Verification items for this drawing (mm, ordinates from the low corner). A direction names the side the tool comes from. Coordinates: 2 decimals unless noted, no trailing zeros. Order: outer loops, then holes, each group sorted by start corner. A loop starts at its lowest first (then second) coordinate and runs counter-clockwise, first axis right, second up. Notation, with made-up numbers: M -39,44 L -35,44 A4 cw -35,51 Z; hole C 53,16.5 d6. An arc over 180 degrees is marked long. One line per item, written item: value. Start each with the question number.
1) Access from +Z, -Z, +X, -X, +Y, -Y to the whole of each face (thin tool, end or side, straight path). Record for the marked faces 4, 5 and 6.
2) Draft check along Y on the marked faces 1, 2 and 3. Enter one of: pulls with the +Y half, pulls with the -Y half, needs draft (parallel to the pull), parting line crosses it, or undercut.
3) Go/stop test with flat-tipped pins: P1, Ø1.6, axis at y = 48, z = 5.5, coming from the -X side; P2, Ø4, axis at y = 41.5, z = 5, coming from the -X side; P3, Ø4.5, axis at x = 13.5, z = 6.5, coming from the +Y side; P4, Ø4, axis at x = 5, y = 28.5, coming from the -Z side. Record where each tip stops, or that it passes through.
4) Sectioned sample at A-A, the plane x = 28. Enter the section's corners in (y, z), then the cut area to 4 significant figures.
5) Sectioned sample at D-D, the plane x = 8. Enter the section's corners in (y, z), then the cut area to 3 significant figures.
6) Sectioned sample at C-C, the plane z = 9.25. Enter the section's corners in (x, y).
7) Sectioned sample at B-B, the plane y = 13. Enter the section's corners in (x, z), then the cut area to 3 significant figures.
8) Thickness scan on L1, parallel to Y at x = 24.5, z = 9.25; L2, parallel to X at y = 12.5, z = 7.25; L3, parallel to Y at x = 9.5, z = 10.5. Record the ranges inside material, lowest first. Write a range as from..to.
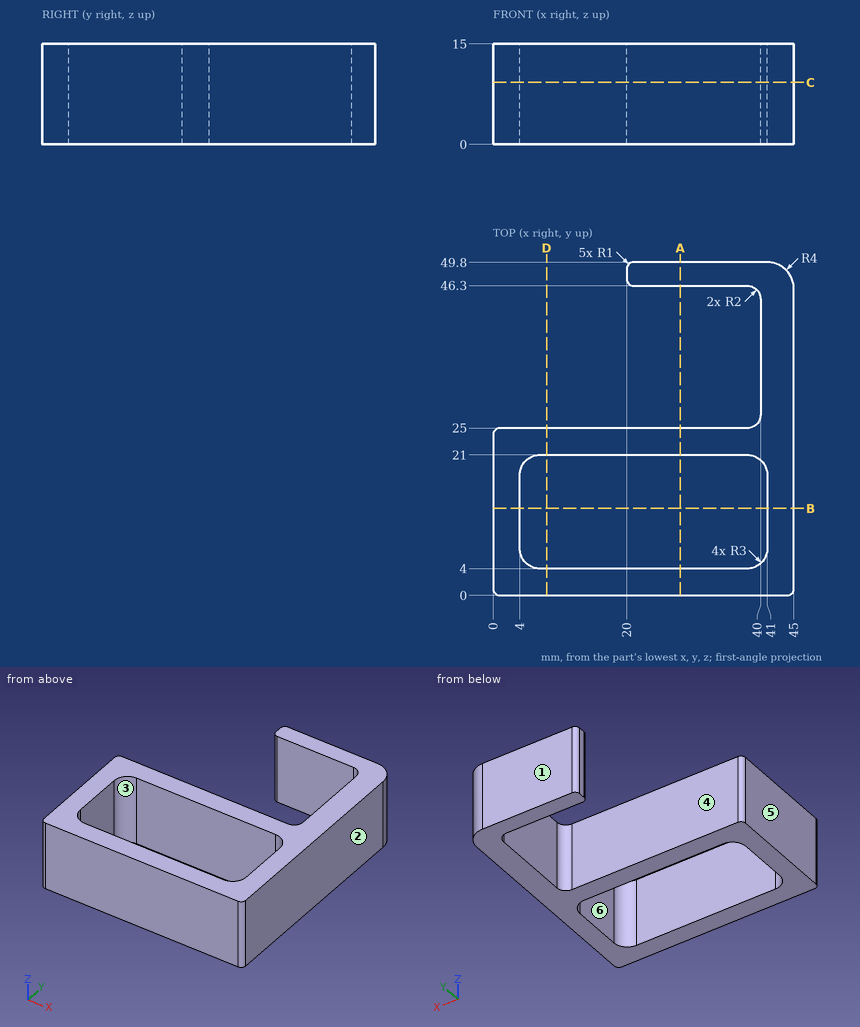
Final values:
1. face 4: +Z, -Z, -X
1. face 5: +Z, -Z, -X, +Y, -Y
1. face 6: +Z, -Z
2. face 1: pulls with the +Y half
2. face 2: needs draft
2. face 3: undercut
3. P1: stops at x = 20
3. P2: stops at x = 40
3. P3: stops at y = 25
3. P4: passes through
4. outline: M 0,0 L 4,0 L 4,15 L 0,15 Z; M 21,0 L 25,0 L 25,15 L 21,15 Z; M 46.3,0 L 49.8,0 L 49.8,15 L 46.3,15 Z
4. area: 172.5 mm^2
5. outline: M 0,0 L 4,0 L 4,15 L 0,15 Z; M 21,0 L 25,0 L 25,15 L 21,15 Z
5. area: 120 mm^2
6. outline: M 0,1 A1 ccw 1,0 L 44,0 A1 ccw 45,1 L 45,45.8 A4 ccw 41,49.8 L 21,49.8 A1 ccw 20,48.8 L 20,47.3 A1 ccw 21,46.3 L 38,46.3 A2 cw 40,44.3 L 40,27 A2 cw 38,25 L 1,25 A1 ccw 0,24 Z; hole M 4,7 A3 ccw 7,4 L 38,4 A3 ccw 41,7 L 41,18 A3 ccw 38,21 L 7,21 A3 ccw 4,18 Z
7. outline: M 0,0 L 4,0 L 4,15 L 0,15 Z; M 41,0 L 45,0 L 45,15 L 41,15 Z
7. area: 120 mm^2
8. L1: y = 0..4, 21..25, 46.3..49.8
8. L2: x = 0..4, 41..45
8. L3: y = 0..4, 21..25
